Answer from the drawing. Dimensions are ordinates in mm from the lowest x, y and z of the part. Give positions to 0.01 mm unless a question says otherwise; leave off trailing zeros. Write each loop counter-clockwise with the first axis right and the second up, starting at its lowest first coordinate (ties: lowest second). Pieces come first, ordered by that corner, then holes.
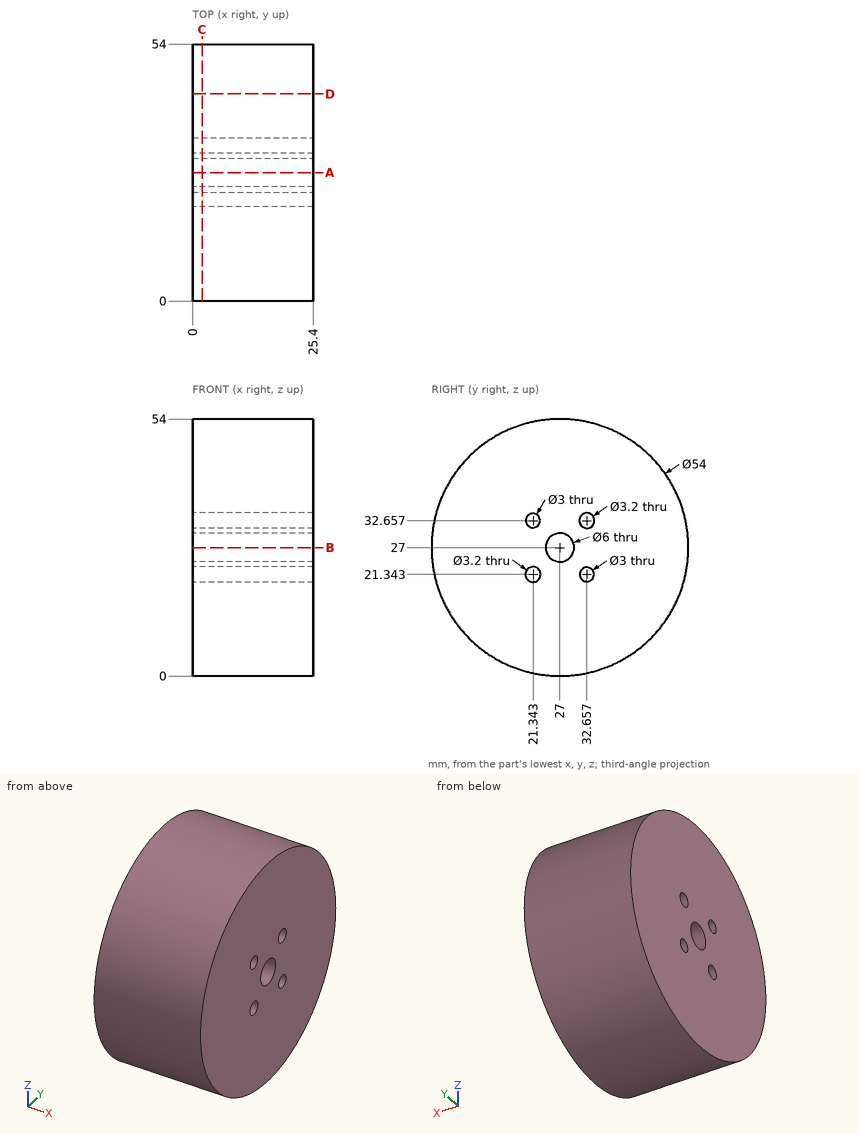
Item 1: Section C-C (x = 2) is taken. Write down the section's boundary in (y, z).
Result set:
outline: circle Ø54 at (27, 27); hole circle Ø3.2 at (21.34, 21.34); hole circle Ø3 at (21.34, 32.66); hole circle Ø6 at (27, 27); hole circle Ø3.2 at (32.66, 32.66); hole circle Ø3 at (32.66, 21.34)
Item 2: Section A-A (y = 27) is taken. Write down the section's boundary in (x, z).
Result set:
outline: (0, 0) - (25.4, 0) - (25.4, 24) - (0, 24) - close; (0, 30) - (25.4, 30) - (25.4, 54) - (0, 54) - close
Item 3: Each of these flat-tipped pins is pushed along its axis until it touches: pin 1 Ø6 at (x, y) = (8.5, 38) entering from +Z; pin 2 Ø1 at (x, y) = (10.5, 45.5) entering from -Z (1 decimal); pin 3 Ø1.5 at (x, y) = (17.5, 7) entering from -Z. Where does it stop, or does it pass through?
Result set:
pin 1: stops at z = 52.79
pin 2: stops at z = 6.9
pin 3: stops at z = 8.07
Item 4: Find the intervals of material crossed by line 1 along Z through (x, y) = (15, 20) (1 decimal); line 2 along Z through (x, y) = (10.75, 27); line 3 along Z through (x, y) = (24.75, 31.5), in increasing order.
Result set:
line 1: z = 0.9 to 20.5, 22.2 to 32, 33.3 to 53.1
line 2: z = 0 to 24, 30 to 54
line 3: z = 0.38 to 20.39, 22.3 to 31.55, 33.76 to 53.62
Item 5: Section D-D (y = 43.5) is taken. Write down the section's boundary in (x, z), and give its area (3 significant figures).
Result set:
outline: (0, 5.63) - (25.4, 5.63) - (25.4, 48.37) - (0, 48.37) - close
area: 1,090 mm2
